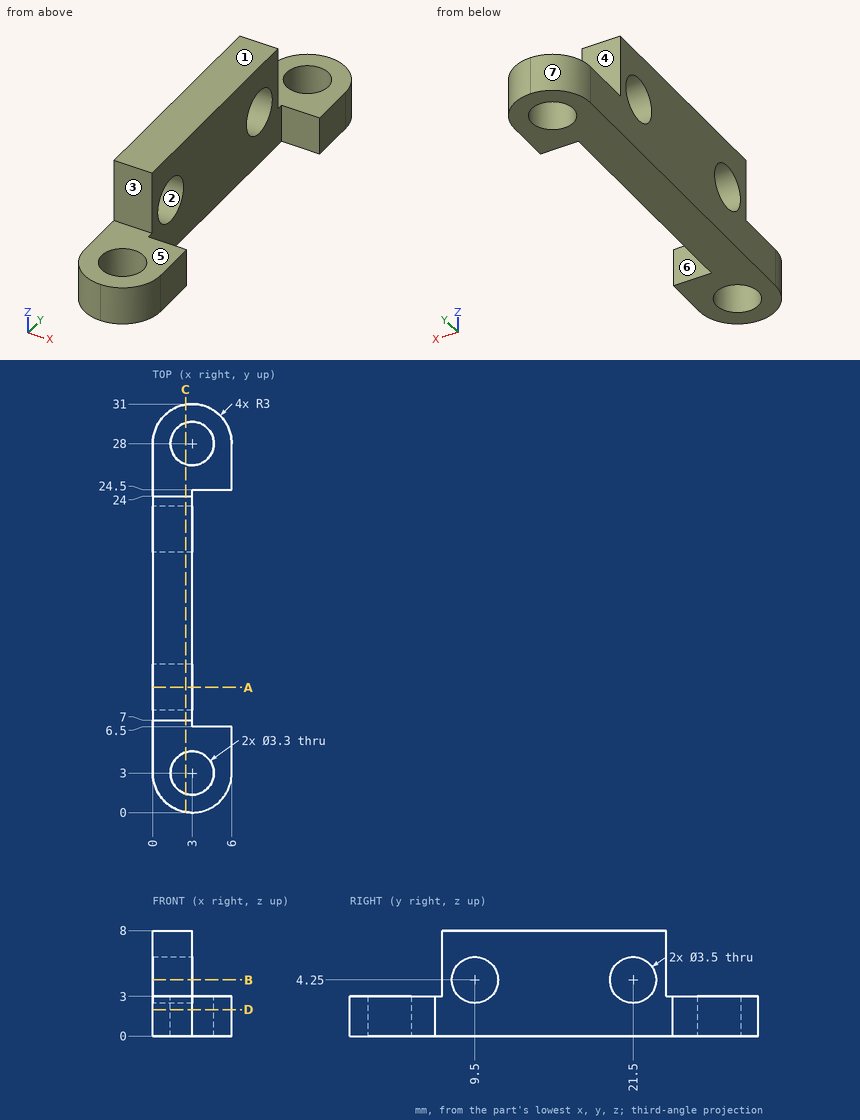
Part print with two shaded views. Sizes in mm from the minimum x, y, z corner. A direction names the side the tool comes from. Round coordinates to 2 decimals unless told otherwise and drop trailing zeros. Order: outer loops, then holes, each group sorted by start corner. A loop starts at its lowest first (then second) coordinate and runs counter-clockwise, first axis right, second up. Notation, with made-up numbers: M 13,76.5 L 28,76.5 A24 ccw 28,94.5 Z; hole C 64.25,55 d2. An arc over 180 degrees is marked long. Answer in a Markdown table with one row per item. Add a question column.
Q1. 3-axis set-ups, long thin cutter, end or side, ignore diameter. For the marked faces 4, 5, 6 and 7: which of +Z, -Z, +X, -X, +Y, -Y reach the whole face in a straight line?
Q2. Cut at D-D on z = 2. Give the number of separate pieces and of enclosed holes in the cut face, and give its area (3 significant figures).
Q3. Cut at B-B on z = 4.25. Give the cut face in (x, y).
Q4. Pin check, flat tips, straight feed: pin 1 (3 mm diameter, centred on x = 4.5, z = 4, fed in from +Y); pin 2 (1 mm diameter, centred on y = 14, z = 6.5, fed in from +X); pin 3 (0.9 mm diameter, centred on x = 5, z = 1, fed in from +Y). Stop position of each tip, or through.
Q5. Wall check: L1, parallel to Y at x = 1.4, z = 4.25; L2, parallel to Y at x = 3.5, z = 1; L3, parallel to X at y = 28, z = 1.95. Give the ranges that are in metal, low to high. Write a range as from..to.
Q6. Cut at C-C on x = 2.5. Give the cut face in (y, z).
Q7. Cut at A-A on y = 9.5. Give the cut face in (x, z), and give its area (3 significant figures).
Q8. Mould opens along Z. For the marked faces 1, 2 and 3 say: +Z half, -Z half, draft (parallel to the pull), parting line (faces both ways), or undercut.
Established:
| question | item | result |
|---|---|---|
| 1 | face 4 | +Z, +X, -X, +Y |
| 1 | face 5 | +Z, +X, -X, -Y |
| 1 | face 6 | +Z, -Z, +X |
| 1 | face 7 | +Z, -Z, -X, +Y |
| 2 | separate pieces | 1 |
| 2 | enclosed holes | 2 |
| 2 | area | 107 mm2 |
| 3 | outline | M 0,7 L 3,7 L 3,7.75 L 0,7.75 Z; M 0,11.25 L 3,11.25 L 3,19.75 L 0,19.75 Z; M 0,23.25 L 3,23.25 L 3,24 L 0,24 Z |
| 4 | pin 1 | stops at y = 30.98 |
| 4 | pin 2 | stops at x = 3 |
| 4 | pin 3 | stops at y = 30.57 |
| 5 | L1 | y = 7..7.75, 11.25..19.75, 23.25..24 |
| 5 | L2 | y = 0.04..1.43, 4.57..6.5, 24.5..26.43, 29.57..30.96 |
| 5 | L3 | x = 0..1.35, 4.65..6 |
| 6 | outline | M 0.04,0 L 1.43,0 L 1.43,3 L 0.04,3 Z; M 4.57,0 L 26.43,0 L 26.43,3 L 24,3 L 24,8 L 7,8 L 7,3 L 4.57,3 Z; M 29.57,0 L 30.96,0 L 30.96,3 L 29.57,3 Z; hole C 9.5,4.25 d3.5; hole C 21.5,4.25 d3.5 |
| 7 | outline | M 0,0 L 3,0 L 3,2.5 L 0,2.5 Z; M 0,6 L 3,6 L 3,8 L 0,8 Z |
| 7 | area | 13.5 mm2 |
| 8 | face 1 | +Z half |
| 8 | face 2 | undercut |
| 8 | face 3 | draft |
